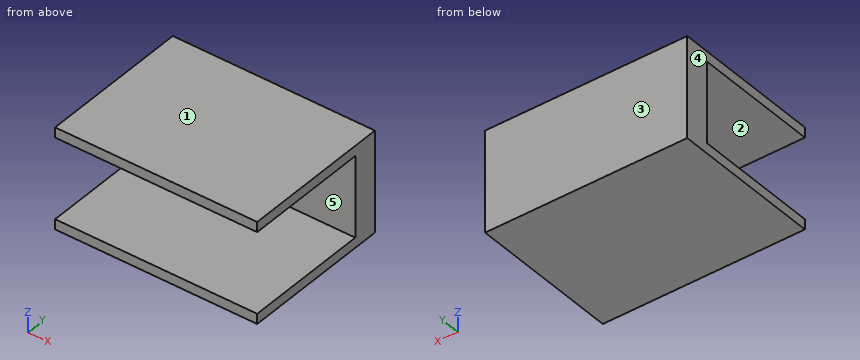
```python
from build123d import *

# Parameters (mm, degrees)
F0_W     = 101.6
F0_H     = 50.8
F1_DEPTH = 76.2
F3_W     = 101.6
F3_H     = 40.64
F4_DEPTH = 63.5


# Not quite as in the source:
# - the program builds the solid bodies; features that only make, move or delete a surface that nothing else refers to are left out


with BuildPart() as f1:
    # F0 (on Front) → F1 (new body)
    with BuildSketch(Plane.XZ):
        with Locations((0.3947839141, -13.1712006897)):
            Rectangle(F0_W, F0_H)
    extrude(amount=-F1_DEPTH)

    # F3 (on face) → F4 (cut)
    with BuildSketch(Plane.XZ):
        with Locations((0.3947839141, -13.1712006897)):
            Rectangle(F3_W, F3_H)
    extrude(amount=-F4_DEPTH, mode=Mode.SUBTRACT)


solid = f1.part
```
Here's how the part is built. I have some questions about the finished solid (model axes, mm). Face numbers are marked on the shaded views. A direction names the side the tool comes from. Give positions to 0.01 mm unless a question says otherwise; leave off trailing zeros. Order: outer loops, then holes, each group sorted by start corner. A loop starts at its lowest first (then second) coordinate and runs counter-clockwise, first axis right, second up. Notation, with made-up numbers: M -1,-35 L 30,-35 A22 ccw 30,-7 Z; hole C 40.25,-21 d8. An arc over 180 degrees is marked long. Use a Markdown table: item, result. Add a question column.
1. Suppose I cut it at A-A (y = 49). List the corners of the cut face in (x, z) for me.
2. Suppose I cut it at C-C (z = -13). List the corners of the cut face in (x, y) for me.
3. I need wall thicknesses on probe 1 along Z at (x, y) = (7.5, 57); probe 2 along Y at (x, z) = (-42.5, -23). Which ranges of each line are inside material? Lowest first, please. Write a range as from..to.
4. If we mould it in two halves opening along Z, with no side actions, what happens to the marked faces 1, 2 and 3? For each: +Z half, -Z half, draft (parallel to the pull), parting line (faces both ways), or undercut.
5. On a 3-axis mill with a long thin cutter (end or side, diameter ignored), from which of +Z, -Z, +X, -X, +Y, -Y can I reach the whole of each face in a straight line? I mean the marked faces 4 and 5. Say none if no direction works.
6. For pin 1 Ø1.5 at (x, z) = (-18, -4.5) entering from -Y; pin 2 Ø10 at (y, z) = (12.5, -27.5) entering from -X, each with a flat end and sliding along its axis, tell me the tip position at first contact or that it passes through.
7. Suppose I cut it at B-B (x = -10). List the corners of the cut face in (y, z) for me.
Results list:
| question | item | result |
|---|---|---|
| 1 | outline | M -50.41,-38.57 L 51.19,-38.57 L 51.19,-33.49 L -50.41,-33.49 Z; M -50.41,7.15 L 51.19,7.15 L 51.19,12.23 L -50.41,12.23 Z |
| 2 | outline | M -50.41,63.5 L 51.19,63.5 L 51.19,76.2 L -50.41,76.2 Z |
| 3 | probe 1 | z = -38.57..-33.49, 7.15..12.23 |
| 3 | probe 2 | y = 63.5..76.2 |
| 4 | face 1 | +Z half |
| 4 | face 2 | undercut |
| 4 | face 3 | draft |
| 5 | face 4 | +Z, -Z, -X, +Y, -Y |
| 5 | face 5 | +X, -X, -Y |
| 6 | pin 1 | stops at y = 63.5 |
| 6 | pin 2 | passes through |
| 7 | outline | M 0,-38.57 L 76.2,-38.57 L 76.2,12.23 L 0,12.23 L 0,7.15 L 63.5,7.15 L 63.5,-33.49 L 0,-33.49 Z |
